from build123d import *

# Parameters (mm, degrees)
SKETCH_1_W               = 19
SKETCH_1_H               = 18
EXTRUDE_1_DEPTH          = 20
EXTRUDE_2_DEPTH          = 5
SKETCH_4_R               = 18.765633517
EXTRUDE_4_DEPTH          = 1
EXTRUDE_5_DEPTH          = 105
SKETCH_12_R              = 18.5
EXTRUDE_13_DEPTH         = 90
SKETCH_13_R              = 3.5
CUT_EXTRUDE_2_DEPTH      = 20
CUT_EXTRUDE_2_DEPTH_BACK = 40
SKETCH_6_R               = 10
CUT_EXTRUDE_3_DEPTH      = 100


with BuildPart() as part:
    # 草图1 → 凸台-拉伸1 (new body)
    with BuildSketch(Plane.XY):
        with Locations((6.777447397, 42.462092888)):
            Rectangle(SKETCH_1_W, SKETCH_1_H)
    extrude(amount=EXTRUDE_1_DEPTH)

    # 草图2 → 凸台-拉伸2 (add)
    with BuildSketch(Plane(origin=(16.277447397, 0, 0), x_dir=(0, 0, -1), z_dir=(1, 0, 0))):
        with BuildLine():
            Line((-29.676018319, 12.462092888), (-29.676018319, 42.462092888))
            Line((-29.676018319, 42.462092888), (-29.676018319, 62.462092888))
            ThreePointArc((-29.676018319, 62.462092888), (-26.747086131, 69.5331607), (-19.676018319, 72.462092888))
            Line((-19.676018319, 72.462092888), (0.323981681, 72.462092888))
            ThreePointArc((0.323981681, 72.462092888), (7.395049493, 69.5331607), (10.323981681, 62.462092888))
            Line((10.323981681, 62.462092888), (10.323981681, 42.462092888))
            Line((10.323981681, 42.462092888), (10.323981681, 12.462092888))
            ThreePointArc((10.323981681, 12.462092888), (-9.676018319, -7.537907112), (-29.676018319, 12.462092888))
        make_face()
    extrude(amount=EXTRUDE_2_DEPTH)

    # 草图4 → 凸台-拉伸4 (add)
    with BuildSketch(Plane(origin=(21.277447397, 0, 0), x_dir=(0, 0, -1), z_dir=(1, 0, 0))):
        with Locations((-9.676018319, 12.462092888)):
            Circle(SKETCH_4_R)
    extrude(amount=EXTRUDE_4_DEPTH)

    # 草图5 → 凸台-拉伸5 (add)
    with BuildSketch(Plane(origin=(21.277447397, 0, 0), x_dir=(0, 0, -1), z_dir=(1, 0, 0))):
        with BuildLine():
            Line((-29.154370976, 52.462092888), (-23.49669222, 67.083579023))
            Line((-23.49669222, 67.083579023), (-16.725326826, 69.463174846))
            Line((-16.725326826, 69.463174846), (-2.765681369, 69.512012284))
            Line((-2.765681369, 69.512012284), (4.144655582, 67.083579023))
            Line((4.144655582, 67.083579023), (9.802334338, 52.462092888))
            ThreePointArc((9.802334338, 52.462092888), (-9.676018319, 32.983740231), (-29.154370976, 52.462092888))
        make_face()
    extrude(amount=EXTRUDE_5_DEPTH)

    # 草图12 → 凸台-拉伸13 (add)
    with BuildSketch(Plane(origin=(0, 51.462092888, 0), x_dir=(1, 0, 0), z_dir=(0, 1, 0))):
        with Locations((41.277447397, -10)):
            Circle(SKETCH_12_R)
    extrude(amount=-EXTRUDE_13_DEPTH)

    # 草图13 → 切除-拉伸2 (cut, two sides)
    with BuildSketch(Plane.XZ.offset(-33.462092888)) as cut_extrude_2_sk:
        with Locations((7.557005132, 10)):
            Circle(SKETCH_13_R)
    extrude(amount=CUT_EXTRUDE_2_DEPTH, mode=Mode.SUBTRACT)
    extrude(cut_extrude_2_sk.sketch, amount=-CUT_EXTRUDE_2_DEPTH_BACK, mode=Mode.SUBTRACT)

    # 草图6 → 切除-拉伸3 (cut)
    with BuildSketch(Plane(origin=(126.277447397, 0, 0), x_dir=(0, 0, -1), z_dir=(1, 0, 0))):
        with Locations((-9.676018319, 52.462092888)):
            Circle(SKETCH_6_R)
    extrude(amount=-CUT_EXTRUDE_3_DEPTH, mode=Mode.SUBTRACT)


solid = part.part
Source: CAD feature listing. Evaluate the final solid. Frame: model axes, mm. A direction names the side the tool comes from. Coordinates: 2 decimals unless noted, no trailing zeros. Loops run counter-clockwise (first coordinate to the right, second up) from the corner with the lowest first, then second, coordinate; pieces in that order, holes last. Notation, with made-up numbers: (34.5, 2) - (55.5, 2) arc R18 ccw to (55.5, 11) - close; hole circle Ø2 at (46.25, 80.25). An arc over 180 degrees is marked (long way). One line per question, with ' | ' between items.
1) Line query: line 1 along X through (y, z) = (14, 10); line 2 along Y through (x, z) = (13, 11); line 3 along Y through (x, z) = (82.5, 10). Output: solid intervals per line, ascending.
Report:
line 1: x = 16.28 to 22.28, 22.78 to 59.78 | line 2: y = 33.46 to 51.46 | line 3: y = 32.99 to 42.47, 62.46 to 69.49
2) Section B-B, the plane y = -2.5. Return loops of the section in (x, z).
Report:
outline: (16.28, -3.6) - (21.28, -3.6) - (21.28, -1.65) - (22.28, -1.65) - (22.28, 21) - (21.28, 21) - (21.28, 22.95) - (16.28, 22.95) - close; circle Ø37 at (41.28, 10)
3) Section C-C, the plane y = 39. Return loops of the section in (x, z).
Report:
outline: (-2.72, 0) - (16.28, 0) - (16.28, -10.32) - (21.28, -10.32) - (21.28, -4.4) - (29.67, -4.4) arc R18.5 ccw to (52.89, -4.4) - (126.28, -4.4) - (126.28, 23.75) - (53.65, 23.75) arc R18.5 ccw to (28.9, 23.75) - (21.28, 23.75) - (21.28, 29.68) - (16.28, 29.68) - (16.28, 20) - (-2.72, 20) - close; hole circle Ø7 at (7.56, 10)
4) First-contact query: P1, Ø9.5, axis at x = 3, z = 10, coming from the -Y side; P2, Ø4, axis at x = 99, z = 21.5, coming from the +Y side; P3, Ø2, axis at x = 44.5, z = 8.5, coming from the +Y side. Flat tips, straight axial feed; report the tip coordinate or a pass-through.
Report:
P1: stops at y = 33.46 | P2: stops at y = 68.49 | P3: stops at y = 69.5
5) Pull-direction query (Y, two-part tool) for faces 4 (the face through (126.277, 43, 5)), 5 (the face through (4.5, 51.462, 7.6)), 6 (the face through (21.277, 32.6, 8.1)); classes: released by +Y, released by -Y, zero draft, split by the parting line, or undercut.
Report:
face 4: zero draft | face 5: released by +Y | face 6: undercut
6) Section A-A, the plane z = 10. Return loops of the section in (x, y), then the cut area to 3 significant figures.
Report:
outline: (-2.72, 33.46) - (4.06, 33.46) - (4.06, 51.46) - (-2.72, 51.46) - close; (11.06, 33.46) - (16.28, 33.46) - (16.28, -7.54) - (21.28, -7.54) - (21.28, -6.3) - (22.28, -6.3) - (22.28, 31.22) - (21.28, 31.22) - (21.28, 32.99) - (22.78, 32.99) - (22.78, -38.54) - (59.78, -38.54) - (59.78, 32.99) - (126.28, 32.99) - (126.28, 42.47) - (26.28, 42.47) - (26.28, 62.46) - (126.28, 62.46) - (126.28, 69.49) - (21.28, 69.49) - (21.28, 72.46) - (16.28, 72.46) - (16.28, 51.46) - (11.06, 51.46) - close | area: 5,130 mm²
7) Set-up query: faces 1 (the face through (22.277, 13, 10)), 2 (the face through (4.5, 33.462, 7.6)), 3 (the face through (18.742, -7.533, 9.236)). Return all of +Z, -Z, +X, -X, +Y, -Y with unobstructed straight access to the full face (end or side cutting, diameter ignored); none if empty.
Report:
face 1: +Z, -Z, -Y | face 2: +Z, -Z, -X, -Y | face 3: -X, -Y
